Input: part model. Units: mm. Frame: model coordinates. A direction names the side the tool comes from. Give positions to 0.01 mm unless a question says otherwise; leave off trailing zeros. Loops run counter-clockwise (first coordinate to the right, second up) from the corner with the lowest first, then second, coordinate; pieces in that order, holes last. Notation, with made-up numbers: M 60.25,31 L 73.25,31 A22 ccw 73.25,54 Z; hole C 82,-29 d6. An arc over 180 degrees is marked long. Use a Markdown table: item, result. Add a question column.
from build123d import *

# Parameters (mm, degrees)
SKETCH1_W           = 1333.4
SKETCH1_H           = 750
BOSS_EXTRUDE1_DEPTH = 80
FILLET1_R           = 20
FILLET2_R           = 20
SKETCH2_R           = 30
SKETCH2_R_2         = 20
BOSS_EXTRUDE2_DEPTH = 750
SKETCH3_R           = 20
CUT_EXTRUDE1_DEPTH  = 750
SKETCH4_R           = 20
BOSS_EXTRUDE3_DEPTH = 10


with BuildPart() as part:
    # Sketch1 → Boss-Extrude1 (new body)
    with BuildSketch(Plane.XY):
        with Locations((-190.485714286, -135.702321429)):
            Rectangle(SKETCH1_W, SKETCH1_H)
    extrude(amount=BOSS_EXTRUDE1_DEPTH)

    # Fillet1
    fillet1_edges = [part.edges().sort_by_distance(p)[0] for p in [
        (-190.485714286, 239.297678571, 0),
    ]]
    fillet(fillet1_edges, radius=FILLET1_R)

    # Fillet2
    fillet2_edges = [part.edges().sort_by_distance(p)[0] for p in [
        (476.214285714, -135.702321429, 80),
        (-857.185714286, -145.702321429, 0),
        (-190.485714286, 239.297678571, 80),
        (476.214285714, 233.439814195, 5.857864376),
        (-857.185714286, 233.439814195, 5.857864376),
        (-857.185714286, -135.702321429, 80),
        (476.214285714, -145.702321429, 0),
        (-190.485714286, -510.702321429, 0),
        (-857.185714286, 239.297678571, 50),
        (476.214285714, 239.297678571, 50),
        (-190.485714286, -510.702321429, 80),
    ]]
    fillet(fillet2_edges, radius=FILLET2_R)

    # Sketch2 → Boss-Extrude2 (add)
    with BuildSketch(Plane(origin=(0, 239.297678571, 0), x_dir=(1, 0, 0), z_dir=(0, 1, 0))):
        with Locations(Location((-876.240324271, -40, 0), (0, 0, 270))):
            Circle(SKETCH2_R)
        with Locations(Location((-876.240324271, -40, 0), (0, 0, 270))):
            Circle(SKETCH2_R_2, mode=Mode.SUBTRACT)
    extrude(amount=-BOSS_EXTRUDE2_DEPTH)

    # Sketch3 → Cut-Extrude1 (cut)
    with BuildSketch(Plane(origin=(0, 239.297678571, 0), x_dir=(1, 0, 0), z_dir=(0, 1, 0))):
        with Locations(Location((-876.240324271, -40, 0), (0, 0, 270))):
            Circle(SKETCH3_R)
    extrude(amount=-CUT_EXTRUDE1_DEPTH, mode=Mode.SUBTRACT)

    # Sketch4 → Boss-Extrude3 (add)
    with BuildSketch(Plane.XY.offset(80)):
        with Locations((-808.393239531, -135.702321429)):
            Circle(SKETCH4_R)
    extrude(amount=BOSS_EXTRUDE3_DEPTH)


solid = part.part
1) Reachability of faces 4 (the cylindrical face through (-789.32, -129.69, 84.93)), 5 (the flat face through (-200, -131, 0)) from +Z, -Z, +X, -X, +Y, -Y: full face, straight path, thin tool, end or side. Return the list, or none.
2) Contact query for flat-ended pins moving along their axis: P1, Ø10, axis at x = -6, z = 75.5, coming from the -Y side; P2, Ø2, axis at y = -101.5, z = 11, coming from the +X side; P3, Ø1, axis at y = -140.5, z = 61.5, coming from the -X side. Output: stop coordinate, or through.
3) Ray query, line 1 (X direction, y = -345, z = 40); line 2 (Y direction, x = -807, z = 61); line 3 (Z direction, x = 110, y = 61.5). Return the intervals inside material, ascending. Write a range as [from, to].
4) Section query B-B, the plane z = 40. Return the cut outline in (x, y), and give its area (3 significant figures).
5) Section query C-C, the plane y = 72. Return the cut outline in (x, z).
6) Section query A-A, the plane x = 13. Return the cut outline in (y, z), and give its area (3 significant figures).
7) Pull-direction query (Z, two-part tool) for faces 1 (the flat face through (-809, -135, 90)), 2 (the cylindrical face through (-856.41, -130.45, 37.4)), 3 (the flat face through (-205, -510.702, 46)); classes: pulls with the +Z half, pulls with the -Z half, needs draft (parallel to the pull), parting line crosses it, or undercut.
Entries:
| question | item | result |
|---|---|---|
| 1 | face 4 | +Z |
| 1 | face 5 | -Z, +X, -X, +Y, -Y |
| 2 | P1 | stops at y = -507.72 |
| 2 | P2 | stops at x = 474.54 |
| 2 | P3 | stops at x = -897.66 |
| 3 | line 1 | x = [-906.24, -896.24], [-856.24, 476.21] |
| 3 | line 2 | y = [-510.68, 239.27] |
| 3 | line 3 | z = [0, 80] |
| 4 | outline | M -906.24,-510.7 L -896.24,-510.7 L -896.24,239.3 L -906.24,239.3 Z; M -856.24,-510.7 L 476.21,-510.7 L 476.21,219.3 A20 ccw 456.21,239.3 L -837.19,239.3 A20 ccw -846.24,237.13 L -846.24,239.3 L -856.24,239.3 Z |
| 4 | area | 1,010,000 mm² |
| 5 | outline | M -856.96,17.01 A20 ccw -837.19,0 L 456.21,0 A20 ccw 476.21,20 L 476.21,60 A20 ccw 456.21,80 L -837.19,80 A20 ccw -856.96,62.99 A30 ccw long Z; hole C -876.24,40 d40 |
| 6 | outline | M -510.7,20 A20 ccw -490.7,0 L 219.3,0 A20 ccw 239.3,20 L 239.3,60 A20 ccw 219.3,80 L -490.7,80 A20 ccw -510.7,60 Z |
| 6 | area | 59,700 mm² |
| 7 | face 1 | pulls with the +Z half |
| 7 | face 2 | undercut |
| 7 | face 3 | needs draft |
